The listing builds one solid part. Answer for the finished solid, in the listing's coordinates (mm). A direction names the side the tool comes from. Round coordinates to 2 decimals unless told otherwise and drop trailing zeros. Write each loop counter-clockwise with the first axis right and the second up, starting at its lowest first coordinate (ties: lowest second). Pieces come first, ordered by that corner, then holes.
(1) For faces 5 (the face through (7, 1, -6)), 6 (the face through (6, -14, 0)), 7 (the face through (4.5, -15, 0)), 8 (the face through (8.5, 0, 1)), 9 (the face through (-4, 16, 5)), determine the directions among +Z, -Z, +X, -X, +Y, -Y from which every point of the face is accessible in a straight line to the end or side of a thin tool.
(2) Find the intervals of material crossed by probe 1 along Y at (x, z) = (6.25, 4.75); probe 2 along X at (y, z) = (30, 0); probe 3 along X at (y, z) = (6.5, 4.5), in increasing order.
(3) A cutting plane is placed at C-C, the plane y = -7. Give the vertices of the cut face in (x, z).
(4) The mould has two halves that part along X. Classify faces 1 (the face through (6.5, 0, 0)), 2 (the face through (-4.88, 33.76, -1.08)), 3 (the face through (-8.5, 0, 1)), 4 (the face through (0, 14, 3)): +X half, -X half, draft (parallel to the pull), parting line (faces both ways), or undercut.
(5) A cutting plane is placed at A-A, the plane z = 0. Give the vertices of the cut face in (x, y).
(6) Each of these flat-tipped pins is pushed along its axis until it touches: pin 1 Ø8 at (x, z) = (0, 0) entering from -Y; pin 2 Ø6.5 at (x, y) = (-2.5, -8) entering from -Z; pin 3 Ø1 at (y, z) = (36, 2) entering from -X. Where does it stop, or does it pass through?
(7) A cutting plane is placed at D-D, the plane y = 30. Give the vertices of the cut face in (x, z).
from build123d import *

# Parameters (mm, degrees)
BOSS_EXTRUDE1_DEPTH = 6
SKETCH2_R           = 5
BOSS_EXTRUDE2_DEPTH = 35
FILLET1_R           = 1
SKETCH3_W           = 17
SKETCH3_H           = 32
BOSS_EXTRUDE3_DEPTH = 1.5
CUT_EXTRUDE1_REACH  = 69.952
SKETCH4_R           = 2.5


with BuildPart() as part:
    # Sketch1 → Boss-Extrude1 (new, symmetric)
    with BuildSketch(Plane.XY):
        Polygon((-6.5, -14), (-6.5, 14), (6.5, 14), (6.5, -14), (4.5, -14), (4.5, -16), (8.5, -16), (8.5, 16), (-8.5, 16), (-8.5, -16), (-4.5, -16), (-4.5, -14), align=None)
    extrude(amount=BOSS_EXTRUDE1_DEPTH, both=True)

    # Sketch2 → Boss-Extrude2 (add)
    with BuildSketch(Plane(origin=(0, 16, 0), x_dir=(1, 0, 0), z_dir=(0, 1, 0))):
        with Locations(Location((0, 0, 0), (0, 0, 270))):
            Circle(SKETCH2_R)
    extrude(amount=BOSS_EXTRUDE2_DEPTH)

    # Fillet1
    fillet1_edges = [part.edges().sort_by_distance(p)[0] for p in [
        (0, 16, -5),
    ]]
    fillet(fillet1_edges, radius=FILLET1_R - 0.0001)  # a hair under: the kernel refuses the full size

    # Sketch3 → Boss-Extrude3 (add)
    with BuildSketch(Plane.XY.offset(6)):
        Rectangle(SKETCH3_W, SKETCH3_H)
    extrude(amount=BOSS_EXTRUDE3_DEPTH)

    # Sketch4 → Cut-Extrude1 (cut, up to next)
    with BuildSketch(Plane(origin=(0, 51, 0), x_dir=(1, 0, 0), z_dir=(0, 1, 0)), mode=Mode.PRIVATE) as cut_extrude1_sk1:
        with Locations(Location((0, 0, 0), (0, 0, 270))):
            Circle(SKETCH4_R)
    cut_extrude1_tool1 = extrude(cut_extrude1_sk1.sketch, amount=-CUT_EXTRUDE1_REACH, mode=Mode.PRIVATE) & part.part
    add(cut_extrude1_tool1.solids().sort_by_distance((0, 51, 0))[0], mode=Mode.SUBTRACT)


solid = part.part
Solutions:
1. face 5: -Z, +X, -X, +Y, -Y
1. face 6: -Z
1. face 7: -Z, -Y
1. face 8: +Z, -Z, +X, +Y, -Y
1. face 9: +Y
2. probe 1: y = -16 to -14, 14 to 16
2. probe 2: x = -5 to -2.5, 2.5 to 5
2. probe 3: x = -8.5 to -6.5, 6.5 to 8.5
3. outline: (-8.5, -6) - (-6.5, -6) - (-6.5, 6) - (6.5, 6) - (6.5, -6) - (8.5, -6) - (8.5, 7.5) - (-8.5, 7.5) - close
4. face 1: undercut
4. face 2: parting line
4. face 3: -X half
4. face 4: undercut
5. outline: (-8.5, -16) - (-4.5, -16) - (-4.5, -14) - (-6.5, -14) - (-6.5, 14) - (-2.5, 14) - (-2.5, 51) - (-5, 51) - (-5, 17) arc R1 cw to (-6, 16) - (-8.5, 16) - close; (2.5, 14) - (6.5, 14) - (6.5, -14) - (4.5, -14) - (4.5, -16) - (8.5, -16) - (8.5, 16) - (6, 16) arc R1 cw to (5, 17) - (5, 51) - (2.5, 51) - close
6. pin 1: stops at y = 14
6. pin 2: stops at z = 6
6. pin 3: stops at x = -4.77
7. outline: circle Ø10 at (0, 0); hole circle Ø5 at (0, 0)
